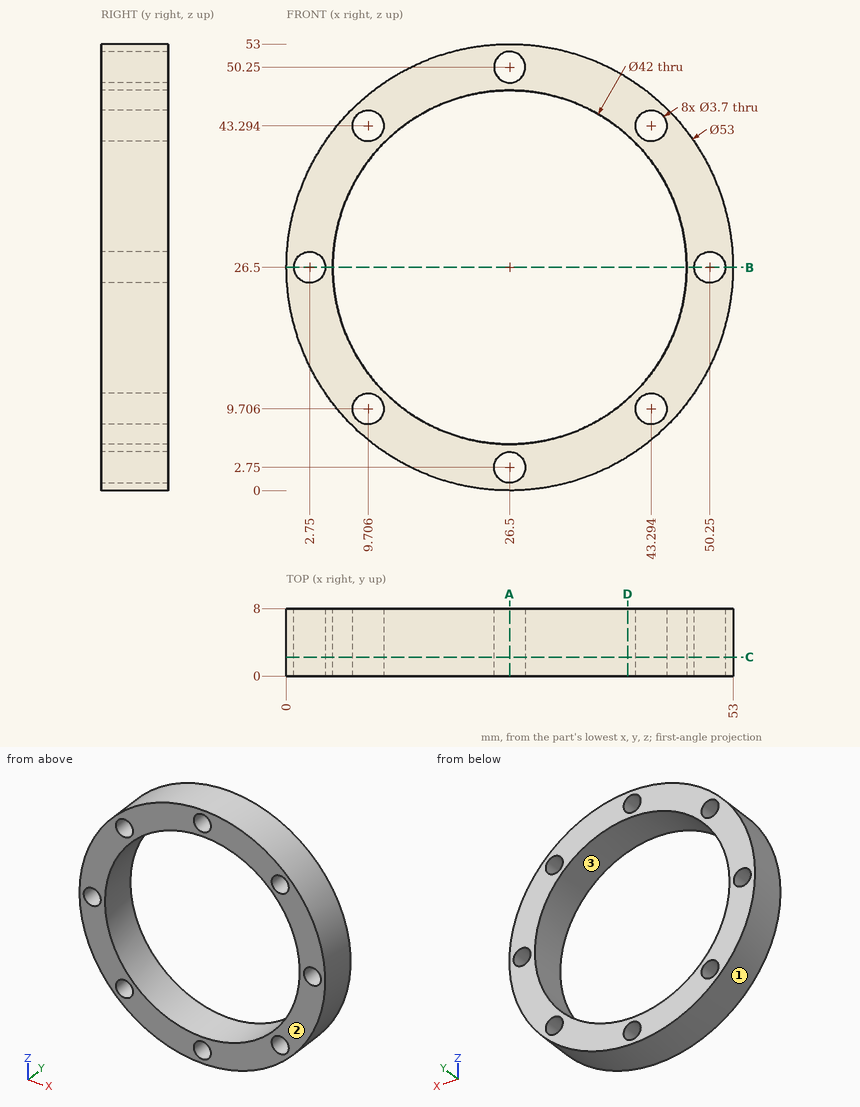
Geometry: see drawing. Coordinates: mm, zero at the bounding-box minimum. Coordinates: 2 decimals unless noted, no trailing zeros. Order: outer loops, then holes, each group sorted by start corner. A loop starts at its lowest first (then second) coordinate and runs counter-clockwise, first axis right, second up. Notation, with made-up numbers: M 18,28.5 L 54,28.5 A23 ccw 54,41.5 Z; hole C 63.25,-31 d8. An arc over 180 degrees is marked long. Answer in a Markdown table with one row per item. Add a question column.
Q1. Section query A-A on x = 26.5. Return the cut outline in (y, z), and give its area (3 significant figures).
Q2. Contact query for flat-ended pins moving along their axis: P1, Ø3.5, axis at x = 2.75, z = 26.5, coming from the +Y side; P2, Ø4, axis at x = 25.5, y = 4, coming from the -Z side; P3, Ø4, axis at x = 39.5, y = 3, coming from the +Z side; P4, Ø4, axis at x = 15.5, y = 3, coming from the +Z side (1 decimal). Output: stop coordinate, or through.
Q3. Section query C-C on y = 2.25. Count the separate pieces of the cut face and the enclosed holes in it, and give its area (3 significant figures).
Q4. Line query: L1, parallel to Z at x = 42.5, y = 0.75 (1 decimal); L2, parallel to Z at x = 38, y = 4 (1 decimal); L3, parallel to X at y = 3.75, z = 10 (1 decimal). Output: solid intervals per line, ascending.
Q5. Mould query, pull axis X, two halves, no side actions, for the marked faces 1, 2 and 3. Classes: released by +X, released by -X, zero draft, split by the parting line, or undercut.
Q6. Section query B-B on z = 26.5. Return the cut outline in (x, y), and give its area (3 significant figures).
Q7. Section query D-D on x = 40.5. Return the cut outline in (y, z).
Completed:
| question | item | result |
|---|---|---|
| 1 | outline | M 0,0 L 8,0 L 8,0.9 L 0,0.9 Z; M 0,4.6 L 8,4.6 L 8,5.5 L 0,5.5 Z; M 0,47.5 L 8,47.5 L 8,48.4 L 0,48.4 Z; M 0,52.1 L 8,52.1 L 8,53 L 0,53 Z |
| 1 | area | 28.8 mm2 |
| 2 | P1 | passes through |
| 2 | P2 | stops at z = 0 |
| 2 | P3 | stops at z = 50.61 |
| 2 | P4 | stops at z = 51.4 |
| 3 | separate pieces | 1 |
| 3 | enclosed holes | 9 |
| 3 | area | 735 mm2 |
| 4 | L1 | z = 5.4 to 8, 11.4 to 12.9, 40.1 to 41.6, 45 to 47.6 |
| 4 | L2 | z = 2.6 to 8.9, 44.1 to 50.4 |
| 4 | L3 | x = 5.8 to 7.9, 11.5 to 13.5, 39.5 to 41.5, 45.1 to 47.2 |
| 5 | face 1 | split by the parting line |
| 5 | face 2 | zero draft |
| 5 | face 3 | undercut |
| 6 | outline | M 0,0 L 0.9,0 L 0.9,8 L 0,8 Z; M 4.6,0 L 5.5,0 L 5.5,8 L 4.6,8 Z; M 47.5,0 L 48.4,0 L 48.4,8 L 47.5,8 Z; M 52.1,0 L 53,0 L 53,8 L 52.1,8 Z |
| 6 | area | 28.8 mm2 |
| 7 | outline | M 0,4 L 8,4 L 8,10.85 L 0,10.85 Z; M 0,42.15 L 8,42.15 L 8,49 L 0,49 Z |
